from build123d import *

# Parameters (mm, degrees)
BOSS_EXTRUDE1_DEPTH = 3
SKETCH2_R           = 5
CUT_EXTRUDE1_DEPTH  = 10
SKETCH4_W           = 3
SKETCH4_H           = 20
BOSS_EXTRUDE3_DEPTH = 3
SKETCH5_R           = 1
CUT_EXTRUDE2_DEPTH  = 10


with BuildPart() as part:
    # Sketch1 → Boss-Extrude1 (new body)
    with BuildSketch(Plane.XY):
        with BuildLine():
            Line((-16.33027103, 11.546525368), (25, 70))
            Line((25, 70), (25, 40))
            Line((25, 40), (19.854388756, -2.408992972))
            ThreePointArc((19.854388756, -2.408992972), (-7.196803073, -18.660279353), (-16.33027103, 11.546525368))
        make_face()
    extrude(amount=-BOSS_EXTRUDE1_DEPTH)

    # Sketch2 → Cut-Extrude1 (cut)
    with BuildSketch(Plane.XY):
        Circle(SKETCH2_R)
    extrude(amount=-CUT_EXTRUDE1_DEPTH, mode=Mode.SUBTRACT)

    # Sketch4 → Boss-Extrude3 (add)
    with BuildSketch(Plane(origin=(25, 0, 0), x_dir=(0, 0, -1), z_dir=(1, 0, 0))):
        with Locations((1.5, 55)):
            Rectangle(SKETCH4_W, SKETCH4_H)
    extrude(amount=BOSS_EXTRUDE3_DEPTH)

    # Sketch5 → Cut-Extrude2 (cut)
    with BuildSketch(Plane.XY):
        with Locations((0, 16.5)):
            Circle(SKETCH5_R)
        with Locations((0, -16.5)):
            Circle(SKETCH5_R)
        with Locations((16.5, 0)):
            Circle(SKETCH5_R)
        with Locations((-16.5, 0)):
            Circle(SKETCH5_R)
    extrude(amount=-CUT_EXTRUDE2_DEPTH, mode=Mode.SUBTRACT)


solid = part.part
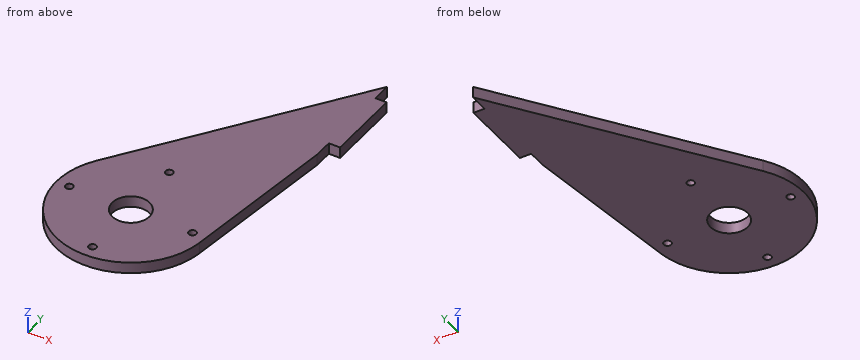
Model file for the job. Use its own axes, mm. Give positions to 0.01 mm unless a question says otherwise; leave off trailing zeros. Order: outer loops, then holes, each group sorted by start corner. A loop starts at its lowest first (then second) coordinate and runs counter-clockwise, first axis right, second up. Notation, with made-up numbers: (61.25, 33.5) -> (112.25, 33.5) arc R16 cw to (112.25, 64.5) -> close; hole circle Ø2 at (58, 69). An arc over 180 degrees is marked (long way). Use CSV: the item, a comma, the result in double quotes.
1. Band-saw the part on D-D, the plane y = 16.5. Give the cut face in (x, z), then the cut area to 3 significant figures.
Outcome:
outline,"(-12.83, -3) -> (-1, -3) -> (-1, 0) -> (-12.83, 0) -> close; (1, -3) -> (22.15, -3) -> (22.15, 0) -> (1, 0) -> close"
area,"98.9 mm²"
2. Drill centre lines: line 1 along Y through (x, z) = (0, -2); line 2 along Y through (x, z) = (-2.5, -0.25); line 3 along Y through (x, z) = (-9, -1.1). Where is each one in solid material? Low to high. Write a range as from..to.
Outcome:
line 1,"-20..-17.5, -15.5..-5, 5..15.5, 17.5..34.64"
line 2,"-19.84..-4.33, 4.33..31.11"
line 3,"-17.86..21.91"
3. Band-saw the part on A-A, the plane x = 0. Give the cut face in (y, z).
Outcome:
outline,"(-20, -3) -> (-17.5, -3) -> (-17.5, 0) -> (-20, 0) -> close; (-15.5, -3) -> (-5, -3) -> (-5, 0) -> (-15.5, 0) -> close; (5, -3) -> (15.5, -3) -> (15.5, 0) -> (5, 0) -> close; (17.5, -3) -> (34.64, -3) -> (34.64, 0) -> (17.5, 0) -> close"
4. Drop flat-ended pins along their axis: pin 1 (1.5 mm diameter, centred on y = -8, z = -1.5, fed in from -X); pin 2 (0.9 mm diameter, centred on y = 42.5, z = -1.5, fed in from +X); pin 3 (6 mm diameter, centred on x = 5.5, y = 35, fed in from +Z); pin 4 (0.9 mm diameter, centred on x = 26, z = -1, fed in from +Y). Give the stop position or say it passes through.
Outcome:
pin 1,"x = -18.64"
pin 2,"x = 25"
pin 3,"z = 0"
pin 4,"y = 65"
5. Band-saw the part on B-B, the plane y = 0. Give the cut face in (x, z).
Outcome:
outline,"(-20, -3) -> (-17.5, -3) -> (-17.5, 0) -> (-20, 0) -> close; (-15.5, -3) -> (-5, -3) -> (-5, 0) -> (-15.5, 0) -> close; (5, -3) -> (15.5, -3) -> (15.5, 0) -> (5, 0) -> close; (17.5, -3) -> (20.15, -3) -> (20.15, 0) -> (17.5, 0) -> close"
6. Band-saw the part on C-C, the plane z = -1.65. Give the cut face in (x, y), then the cut area to 3 significant figures.
Outcome:
outline,"(-16.33, 11.55) arc R20 ccw (long way) to (19.85, -2.41) -> (25, 40) -> (25, 45) -> (28, 45) -> (28, 65) -> (25, 65) -> (25, 70) -> close; hole circle Ø2 at (-16.5, 0); hole circle Ø10 at (0, 0); hole circle Ø2 at (0, -16.5); hole circle Ø2 at (0, 16.5); hole circle Ø2 at (16.5, 0)"
area,"2,210 mm²"
